```python
from build123d import *

# Parameters (mm, degrees)
SKETCH1_W                      = 150
SKETCH1_H                      = 335
BASE_FLANGE1_DEPTH             = 2
EDGE_FLANGE1_STRIP_W           = 13
EDGE_FLANGE1_STRIP_H           = 2
EDGE_FLANGE1_STRIP_CUT_DEPTH   = 335
EDGE_FLANGE1_STRIP_2_W         = 13
EDGE_FLANGE1_STRIP_2_H         = 2
EDGE_FLANGE1_STRIP_CUT_2_DEPTH = 335
EDGE_FLANGE1_DEPTH             = 335
EDGE_FLANGE1_BEND_DEPTH        = 335
SKETCH11_W                     = 86
SKETCH11_H                     = 30
CUT_EXTRUDE1_DEPTH             = 10


# Sheet-metal steps are written as plain solids
with BuildPart() as part:
    # Sketch1 → Base-Flange1 (new body)
    with BuildSketch(Plane(origin=(0, 0, 0), x_dir=(0, 0, -1), z_dir=(1, 0, 0))):
        Rectangle(SKETCH1_W, SKETCH1_H)
    extrude(amount=-BASE_FLANGE1_DEPTH)

    # Edge-Flange1 strip (across the edge) → Edge-Flange1 strip cut (cut)
    with BuildSketch(Plane(origin=(0, -167.5, -75), x_dir=(0, 0, 1), z_dir=(0, 1, 0))):
        with Locations((-2, -1)):
            Rectangle(EDGE_FLANGE1_STRIP_W, EDGE_FLANGE1_STRIP_H)
    extrude(amount=EDGE_FLANGE1_STRIP_CUT_DEPTH, mode=Mode.SUBTRACT)

    # Edge-Flange1 strip 2 (across the edge) → Edge-Flange1 strip cut 2 (cut)
    with BuildSketch(Plane(origin=(0, 167.5, 75), x_dir=(0, 0, -1), z_dir=(0, -1, 0))):
        with Locations((-2, -1)):
            Rectangle(EDGE_FLANGE1_STRIP_2_W, EDGE_FLANGE1_STRIP_2_H)
    extrude(amount=EDGE_FLANGE1_STRIP_CUT_2_DEPTH, mode=Mode.SUBTRACT)

    # Edge-Flange1 section (across the edge) → Edge-Flange1 (add)
    with BuildSketch(Plane(origin=(0, -167.5, -75), x_dir=(0, 0, 1), z_dir=(0, 1, 0))):
        with BuildLine():
            Line((0, 2.5), (0, 26))
            Line((0, 26), (2, 26))
            Line((2, 26), (2, 2.5))
            ThreePointArc((2, 2.5), (2.732233047, 0.732233047), (4.5, 0))
            Line((4.5, 0), (4.5, -2))
            ThreePointArc((4.5, -2), (1.318019485, -0.681980515), (0, 2.5))
        make_face()
    extrude(amount=EDGE_FLANGE1_DEPTH)

    # Edge-Flange1 section 2 (across the edge) → Edge-Flange1 bend (add)
    with BuildSketch(Plane(origin=(0, 167.5, 75), x_dir=(0, 0, -1), z_dir=(0, -1, 0))):
        with BuildLine():
            Line((0, 2.5), (0, 26))
            Line((0, 26), (2, 26))
            Line((2, 26), (2, 2.5))
            ThreePointArc((2, 2.5), (2.732233047, 0.732233047), (4.5, 0))
            Line((4.5, 0), (4.5, -2))
            ThreePointArc((4.5, -2), (1.318019485, -0.681980515), (0, 2.5))
        make_face()
    extrude(amount=EDGE_FLANGE1_BEND_DEPTH)

    # Sketch11 → Cut-Extrude1 (cut)
    with BuildSketch(Plane(origin=(0, 0, 0), x_dir=(0, 0, -1), z_dir=(1, 0, 0))):
        with Locations((0, 152.5)):
            Rectangle(SKETCH11_W, SKETCH11_H)
    cut_extrude1 = extrude(amount=-CUT_EXTRUDE1_DEPTH, mode=Mode.SUBTRACT)

    # Mirror1: Cut-Extrude1 across plane
    add(cut_extrude1.mirror(Plane.ZX), mode=Mode.SUBTRACT)


solid = part.part
```
Could you check a few things on this model? Use its own coordinates, in mm. A direction names the side the tool comes from. Coordinates: 2 decimals unless noted, no trailing zeros. Order: outer loops, then holes, each group sorted by start corner. A loop starts at its lowest first (then second) coordinate and runs counter-clockwise, first axis right, second up. Notation, with made-up numbers: M 74,-16 L 133,-16 A22 cw 133,-5 Z; hole C 51,85.5 d2. An arc over 180 degrees is marked long. Use one line per item in the form item = value. Start each with the question number.
1. Suppose I cut it at D-D on z = 32.5. Write out the boundary of the cut face in (x, y), then the cut area to 3 significant figures.
2. On a 3-axis mill with a long thin cutter (end or side, diameter ignored), from which of +Z, -Z, +X, -X, +Y, -Y can I reach the whole of each face in a straight line? I mean faces 5 (the flat face through (0, 2, 1)), 6 (the flat face through (-2, 2, 1)). Say none if no direction works.
3. Suppose I cut it at B-B on y = 112.5. Write out the boundary of the cut face in (x, z).
4. Suppose I cut it at C-C on z = -64.5. Write out the boundary of the cut face in (x, y).
5. For pin 1 (2 mm diameter, centred on x = -0.5, z = -5.5, fed in from +Y); pin 2 (1.6 mm diameter, centred on x = -0.5, y = 151.5, fed in from +Z); pin 3 (0.6 mm diameter, centred on x = -1, y = -153.5, fed in from -Z), each with a flat end and sliding along its axis, tell me the tip position at first contact or that it passes through.
6. We'd pull the mould along Z, two halves only. Please class faces 1 (the flat face through (-0.4, 167.5, 66)), 2 (the flat face through (14, 2, 73)), 3 (the flat face through (14, 2, 75)), 4 (the flat face through (14, -2, -73)): +Z half, -Z half, draft (parallel to the pull), parting line (faces both ways), or undercut.
7. Suppose I cut it at A-A on x = 16.5. Write out the boundary of the cut face in (y, z).
8. Please list where these lines run through material, in increasing order: line 1 (Z direction, x = 2.25, y = -28); line 2 (X direction, y = -20.5, z = 27); line 3 (Z direction, x = -0.5, y = -130).
Geometry says:
q1.outline = M -2,-137.5 L 0,-137.5 L 0,137.5 L -2,137.5 Z
q1.area = 550 mm^2
q2.face_5 = +X, +Y, -Y
q2.face_6 = +Z, -Z, -X, +Y, -Y
q3.outline = M -2,-70.5 A4.5 ccw 2.5,-75 L 26,-75 L 26,-73 L 2.5,-73 A2.5 cw 0,-70.5 L 0,70.5 A2.5 cw 2.5,73 L 26,73 L 26,75 L 2.5,75 A4.5 ccw -2,70.5 Z
q4.outline = M -2,-167.5 L 0,-167.5 L 0,167.5 L -2,167.5 Z
q5.pin_1 = 137.5
q5.pin_2 = 74.43
q5.pin_3 = -73.66
q6.face_1 = draft
q6.face_2 = undercut
q6.face_3 = +Z half
q6.face_4 = undercut
q7.outline = M -167.5,-75 L 167.5,-75 L 167.5,-73 L -167.5,-73 Z; M -167.5,73 L 167.5,73 L 167.5,75 L -167.5,75 Z
q8.line_1 = -74.99 to -72.99, 72.99 to 74.99
q8.line_2 = -2 to 0
q8.line_3 = -73.85 to 73.85
